Source: CAD feature listing. Evaluate the final solid. Frame: model axes, mm. Round coordinates to 2 decimals unless told otherwise and drop trailing zeros. Loops run counter-clockwise (first coordinate to the right, second up) from the corner with the lowest first, then second, coordinate; pieces in that order, holes last. Notation, with made-up numbers: M 22.25,86 L 50.25,86 A22 ccw 50.25,106 Z; hole C 12.5,12.5 d4. An arc over 180 degrees is marked long. One line per item, written item: value.
from build123d import *

# Parameters (mm, degrees)
SKETCH1_R           = 1.55
BOSS_EXTRUDE1_DEPTH = 2
CHAMFER1_SIZE       = 0.1


with BuildPart() as part:
    # Sketch1 → Boss-Extrude1 (new body)
    with BuildSketch(Plane.XY):
        with BuildLine():
            Line((-11.929744939, 2.5), (12.070255061, 2.5))
            ThreePointArc((12.070255061, 2.5), (14.570255061, 0), (12.070255061, -2.5))
            Line((12.070255061, -2.5), (-11.929744939, -2.5))
            ThreePointArc((-11.929744939, -2.5), (-14.429744939, 0), (-11.929744939, 2.5))
        make_face()
        with Locations((12.070255061, 0)):
            Circle(SKETCH1_R, mode=Mode.SUBTRACT)
        with Locations((-11.929744939, 0)):
            Circle(SKETCH1_R, mode=Mode.SUBTRACT)
    extrude(amount=BOSS_EXTRUDE1_DEPTH)

    # Chamfer1
    chamfer1_edges = [part.edges().sort_by_distance(p)[0] for p in [
        (14.570255061, 0, 2),
        (0.070255061, 2.5, 2),
        (-14.429744939, 0, 2),
        (0.070255061, 2.5, 0),
        (14.570255061, 0, 0),
        (0.070255061, -2.5, 0),
        (-14.429744939, 0, 0),
        (0.070255061, -2.5, 2),
    ]]
    chamfer(chamfer1_edges, length=CHAMFER1_SIZE)


solid = part.part
1. Section query A-A (y = 0). Return the cut outline in (x, z).
Report:
outline: M -14.43,0.1 L -14.33,0 L -13.48,0 L -13.48,2 L -14.33,2 L -14.43,1.9 Z; M -10.38,0 L 10.52,0 L 10.52,2 L -10.38,2 Z; M 13.62,0 L 14.47,0 L 14.57,0.1 L 14.57,1.9 L 14.47,2 L 13.62,2 Z
2. Ray query, line 1 (X direction, y = -0.2, z = 1.3); line 2 (X direction, y = -0.5, z = 1.4); line 3 (Y direction, x = 12.5, z = 1.1). Return the intervals inside material, ascending. Write a range as [from, to].
Report:
line 1: x = [-14.42, -13.47], [-10.39, 10.53], [13.61, 14.56]
line 2: x = [-14.38, -13.4], [-10.46, 10.6], [13.54, 14.52]
line 3: y = [-2.46, -1.49], [1.49, 2.46]
3. Pin query (flat end, axial travel): pin 1 (3 mm diameter, centred on x = -11.93, y = 0, fed in from +Z). Return the tip coordinate at first contact, or that it passes through.
Report:
pin 1: passes through
4. Section query B-B (z = 0.4). Return the cut outline in (x, y), and give its area (3 significant figures).
Report:
outline: M -11.93,-2.5 L 12.07,-2.5 A2.5 ccw 12.07,2.5 L -11.93,2.5 A2.5 ccw Z; hole C -11.93,0 d3.1; hole C 12.07,0 d3.1
area: 125 mm2
5. Pull-direction query (X, two-part tool) for faces 1 (the face through (14.57, 0.05, 0.99)), 2 (the face through (-14.43, -0.05, 0.99)), 3 (the face through (-10.451, 0.466, 0.986)), 4 (the face through (0, 2.5, 1)); classes: released by +X, released by -X, zero draft, split by the parting line, or undercut.
Report:
face 1: released by +X
face 2: released by -X
face 3: undercut
face 4: zero draft
